Check sheet for the modelled part. Datum: model origin and axes. Units: mm. A direction names the side the tool comes from. Give positions to 0.01 mm unless a question says otherwise; leave off trailing zeros. Loops run counter-clockwise (first coordinate to the right, second up) from the corner with the lowest first, then second, coordinate; pieces in that order, holes last. Notation, with made-up numbers: M 15.5,31.5 L 58.5,31.5 A34 cw 58.5,68.5 Z; hole C 4,-19 d2. An arc over 180 degrees is marked long. Write each question's results on one line, items separated by ' | '. Start each with the question number.
1. Sectioned sample at D-D on z = -10. Record the cut outline in (x, y).
2. Go/stop test with flat-tipped pins: pin 1 (1 mm diameter, centred on y = -10, z = -9, fed in from -X); pin 2 (10 mm diameter, centred on y = -12, z = -55.5, fed in from -X); pin 3 (2 mm diameter, centred on y = 34.5, z = -18.5, fed in from +X). Record where each tip stops, or that it passes through.
3. Tool access check on faces 4 (the cylindrical face through (-11.056, -49.787, -74.65)), 5 (the flat face through (16, -49, -100)). Record the directions out of +Z, -Z, +X, -X, +Y, -Y that give a thin tool (end or side, any length) a straight path to the whole face; none if there is none.
4. Draft check along X on faces 1 (the cylindrical face through (-11.923, -53.692, -51.835)), 2 (the flat face through (-1, 1, 5)), 3 (the flat face through (-1, 1, 0)). Enter one of: pulls with the +X half, pulls with the -X half, needs draft (parallel to the pull), parting line crosses it, or undercut.
5. Material ranges on line 1 along Y through (x, z) = (0, -27); line 2 along Y through (x, z) = (0, -65.5); line 3 along X through (y, z) = (1, -81.5), recorded low to high.
6. Sectioned sample at B-B on z = -69. Record the cut outline in (x, y).
7. Sectioned sample at A-A on x = 0. Record the cut outline in (y, z).
```python
from build123d import *

# Parameters (mm, degrees)
F0_R     = 55
F0_R_2   = 51
F0_R_3   = 47
F1_DEPTH = 5
F2_DEPTH = 50
F3_DEPTH = 100
F4_R     = 10


with BuildPart() as f1:
    # F0 (on Top) → F1 (new body)
    with BuildSketch(Plane.XY):
        Circle(F0_R)
        Circle(F0_R_2, mode=Mode.SUBTRACT)
        Circle(F0_R_2)
        Circle(F0_R_3, mode=Mode.SUBTRACT)
        Circle(F0_R_3)
    extrude(amount=F1_DEPTH)

    # F0 (on Top) → F2 (join)
    with BuildSketch(Plane.XY):
        Circle(F0_R_2)
        Circle(F0_R_3, mode=Mode.SUBTRACT)
    extrude(amount=-F2_DEPTH)

    # F0 (on Top) → F3 (join)
    with BuildSketch(Plane.XY):
        Circle(F0_R)
        Circle(F0_R_2, mode=Mode.SUBTRACT)
    extrude(amount=-F3_DEPTH)

    # F4
    f4_edges = [f1.edges().sort_by_distance(p)[0] for p in [
        (-55, 0, 5),
    ]]
    fillet(f4_edges, radius=F4_R)


solid = f1.part
```
Output values:
1) outline: C 0,0 d110; hole C 0,0 d94
2) pin 1: x = -54.17 | pin 2: x = -54.55 | pin 3: x = 43.62
3) face 4: -Z | face 5: -Z, +X, -X, +Y, -Y
4) face 1: parting line crosses it | face 2: needs draft | face 3: undercut
5) line 1: -55 to -47, 47 to 55 | line 2: -55 to -51, 51 to 55 | line 3: -54.99 to -50.99, 50.99 to 54.99
6) outline: C 0,0 d110; hole C 0,0 d102
7) outline: M -55,-100 L -51,-100 L -51,-50 L -47,-50 L -47,0 L 47,0 L 47,-50 L 51,-50 L 51,-100 L 55,-100 L 55,-5 A10 ccw 45,5 L -45,5 A10 ccw -55,-5 Z
